Read the model definition and answer for the solid it produces. Units are mm, in the model's axes. Round coordinates to 2 decimals unless told otherwise and drop trailing zeros. Order: outer loops, then holes, each group sorted by start corner. A loop starts at its lowest first (then second) coordinate and runs counter-clockwise, first axis right, second up. Notation, with made-up numbers: (11, 55.5) -> (54, 55.5) arc R23 ccw to (54, 65.5) -> close; hole circle Ø10 at (-25, 4.5). An arc over 180 degrees is marked (long way). One line per item, written item: value. Start each with the question number.
1. A flat-ended cylindrical pin translates along its axis: pin 1 Ø0.9 at (x, y) = (55.5, 2) entering from +Z. Find the tip coordinate at first contact, or state that the pin passes through.
2. Section C-C (y = 2) is taken. Give the vertices of the cut face in (x, z), then the cut area to 3 significant figures.
3. Consider line 1 (X direction, y = 1.35, z = -50.5); line 2 (Z direction, x = 33, y = 1.2); line 3 (X direction, y = 0.6, z = -53). Determine where each line is inside the solid, lowest interval first.
4. Section B-B (x = 25.5) is taken. Give the vertices of the cut face in (y, z), then the cut area to 3 significant figures.
5. Section A-A (z = -61.5) is taken. Give the vertices of the cut face in (x, y).
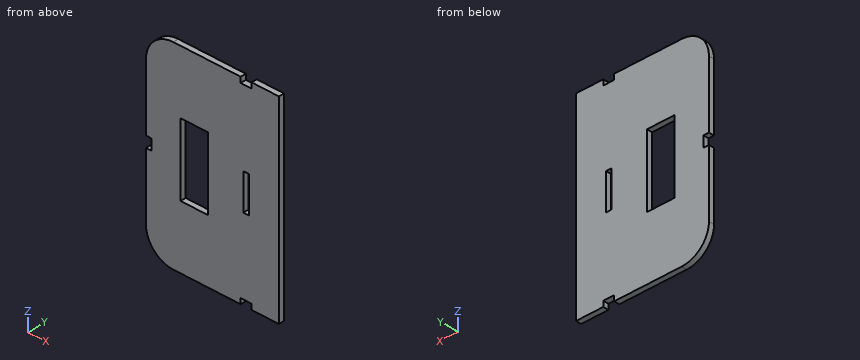
from build123d import *

# Parameters (mm, degrees)
EXTRUDE_3_DEPTH    = 3
SKETCH1_W          = 15
SKETCH1_H          = 40
SKETCH1_W_2        = 3
SKETCH1_H_2        = 20
CUT_EXTRUDE1_DEPTH = 10
FILLET1_R          = 15


with BuildPart() as part:
    # Эскиз4 → Бобышка-Вытянуть3 (new body)
    with BuildSketch(Plane(origin=(0, 0, 0), x_dir=(1, 0, 0), z_dir=(0, 1, 0))):
        Polygon((0, 110), (0, 58), (3, 58), (3, 52), (0, 52), (0, 0), (52, 0), (52, 3), (58, 3), (58, 0), (73, 0), (73, 110), (58, 110), (58, 107), (52, 107), (52, 110), align=None)
    extrude(amount=EXTRUDE_3_DEPTH)

    # Sketch1 → Cut-Extrude1 (cut)
    with BuildSketch(Plane(origin=(0, 3, 0), x_dir=(1, 0, 0), z_dir=(0, 1, 0))):
        with Locations((26.5, 55)):
            Rectangle(SKETCH1_W, SKETCH1_H)
        with Locations((55, 55)):
            Rectangle(SKETCH1_W_2, SKETCH1_H_2)
    extrude(amount=-CUT_EXTRUDE1_DEPTH, mode=Mode.SUBTRACT)

    # Fillet1
    fillet1_edges = [part.edges().sort_by_distance(p)[0] for p in [
        (0, 1.5, 0),
        (0, 1.5, -110),
    ]]
    fillet(fillet1_edges, radius=FILLET1_R)


solid = part.part
Answer:
1. pin 1: z = -3
2. outline: (0, -95) arc R15 ccw to (15, -110) -> (52, -110) -> (52, -107) -> (58, -107) -> (58, -110) -> (73, -110) -> (73, 0) -> (58, 0) -> (58, -3) -> (52, -3) -> (52, 0) -> (15, 0) arc R15 ccw to (0, -15) -> (0, -52) -> (3, -52) -> (3, -58) -> (0, -58) -> close; hole (19, -75) -> (34, -75) -> (34, -35) -> (19, -35) -> close; hole (53.5, -65) -> (56.5, -65) -> (56.5, -45) -> (53.5, -45) -> close
2. area: 7,220 mm^2
3. line 1: 0 to 19, 34 to 53.5, 56.5 to 73
3. line 2: -110 to -75, -35 to 0
3. line 3: 3 to 19, 34 to 53.5, 56.5 to 73
4. outline: (0, -110) -> (3, -110) -> (3, -75) -> (0, -75) -> close; (0, -35) -> (3, -35) -> (3, 0) -> (0, 0) -> close
4. area: 210 mm^2
5. outline: (0, 0) -> (19, 0) -> (19, 3) -> (0, 3) -> close; (34, 0) -> (53.5, 0) -> (53.5, 3) -> (34, 3) -> close; (56.5, 0) -> (73, 0) -> (73, 3) -> (56.5, 3) -> close
